```python
from build123d import *

# Parameters (mm, degrees)
BASE_W_MOTOR_MOUNTS_R     = 70
BASE_W_MOTOR_MOUNTS_R_2   = 1.651
BOSS_EXTRUDE1_DEPTH       = 3.175
STANDOFFS_TOP_BOTTOM_R    = 1.65
CUT_EXTRUDE2_DEPTH        = 3.175
PI_AND_MEGA_STANDOFFS_R   = 1.4
PI_AND_MEGA_STANDOFFS_R_2 = 1.65
CUT_EXTRUDE3_DEPTH        = 3.175


with BuildPart() as part:
    # Base w/ Motor Mounts → Boss-Extrude1 (new body)
    with BuildSketch(Plane(origin=(0, 0, 0), x_dir=(1, 0, 0), z_dir=(0, 1, 0))):
        Circle(BASE_W_MOTOR_MOUNTS_R)
        with Locations((44.55, 0)):
            Circle(BASE_W_MOTOR_MOUNTS_R_2, mode=Mode.SUBTRACT)
        with Locations((54.075, 10.85)):
            Circle(BASE_W_MOTOR_MOUNTS_R_2, mode=Mode.SUBTRACT)
        with Locations((54.075, -10.85)):
            Circle(BASE_W_MOTOR_MOUNTS_R_2, mode=Mode.SUBTRACT)
        with Locations((-54.075, -10.85)):
            Circle(BASE_W_MOTOR_MOUNTS_R_2, mode=Mode.SUBTRACT)
        with Locations((-54.075, 10.85)):
            Circle(BASE_W_MOTOR_MOUNTS_R_2, mode=Mode.SUBTRACT)
        with Locations((-44.55, 0)):
            Circle(BASE_W_MOTOR_MOUNTS_R_2, mode=Mode.SUBTRACT)
    extrude(amount=BOSS_EXTRUDE1_DEPTH)

    # Standoffs (top / bottom) → Cut-Extrude2 (cut)
    with BuildSketch(Plane(origin=(0, 0, 0), x_dir=(1, 0, 0), z_dir=(0, 1, 0))):
        with Locations((60.976049146, 25.257106536)):
            Circle(STANDOFFS_TOP_BOTTOM_R)
        with Locations((60.976049146, -25.257106536)):
            Circle(STANDOFFS_TOP_BOTTOM_R)
        with Locations((-60.976049146, -25.257106536)):
            Circle(STANDOFFS_TOP_BOTTOM_R)
        with Locations((-60.976049146, 25.257106536)):
            Circle(STANDOFFS_TOP_BOTTOM_R)
        with Locations((35, 48.621778265)):
            Circle(STANDOFFS_TOP_BOTTOM_R)
        with Locations((35, 30.621778265)):
            Circle(STANDOFFS_TOP_BOTTOM_R)
        with Locations((35, -30.621778265)):
            Circle(STANDOFFS_TOP_BOTTOM_R)
        with Locations((35, -48.621778265)):
            Circle(STANDOFFS_TOP_BOTTOM_R)
        with Locations((-35, -48.621778265)):
            Circle(STANDOFFS_TOP_BOTTOM_R)
        with Locations((-35, -30.621778265)):
            Circle(STANDOFFS_TOP_BOTTOM_R)
        with Locations((-35, 30.621778265)):
            Circle(STANDOFFS_TOP_BOTTOM_R)
        with Locations((-35, 48.621778265)):
            Circle(STANDOFFS_TOP_BOTTOM_R)
    extrude(amount=CUT_EXTRUDE2_DEPTH, mode=Mode.SUBTRACT)

    # Pi and Mega Standoffs → Cut-Extrude3 (cut)
    with BuildSketch(Plane(origin=(0, 0, 0), x_dir=(1, 0, 0), z_dir=(0, 1, 0))):
        with Locations((-19.9, 55)):
            Circle(PI_AND_MEGA_STANDOFFS_R)
        with Locations((38.1, 55)):
            Circle(PI_AND_MEGA_STANDOFFS_R)
        with Locations((38.1, 6)):
            Circle(PI_AND_MEGA_STANDOFFS_R)
        with Locations((-19.9, 6)):
            Circle(PI_AND_MEGA_STANDOFFS_R)
        with Locations((-38.1, -54.2)):
            Circle(PI_AND_MEGA_STANDOFFS_R_2)
        with Locations((-36.8, -6)):
            Circle(PI_AND_MEGA_STANDOFFS_R_2)
        with Locations((38.1, -6)):
            Circle(PI_AND_MEGA_STANDOFFS_R_2)
    extrude(amount=CUT_EXTRUDE3_DEPTH, mode=Mode.SUBTRACT)


solid = part.part
```
Design review of the part built by this model. Coordinates are the model's own, in mm. Coordinates: 2 decimals unless noted, no trailing zeros. Order: outer loops, then holes, each group sorted by start corner. A loop starts at its lowest first (then second) coordinate and runs counter-clockwise, first axis right, second up. Notation, with made-up numbers: M 7,48.25 L 19,48.25 A19 ccw 19,76.25 Z; hole C -23,-11.75 d10. An arc over 180 degrees is marked long. Answer as a JSON object with one key per item and string values. Group by question number.
1) For pin 1 (1 mm diameter, centred on y = 1, z = -53.5, fed in from +X), flat-tipped, find the tip position at first contact; note if it passes through.
2) Wall thickness on L1, parallel to Z at x = -19.9, y = 2.5; L2, parallel to Z at x = -35, y = 1.6; L3, parallel to Z at x = 37, y = 0.9: over which ranges is each line inside the solid? List them lowest first.
3) Add section D-D, the plane x = -24.5. Write out the cut boundary in (y, z) (3 decimals).
4) Add section C-C, the plane x = -44.55. Write out the cut boundary in (y, z) (1 decimal), then the cut area to 3 significant figures.
5) Add section B-B, the plane y = 2.25. Count the separate pieces of the cut face and the enclosed holes in it, then the cut area to 3 significant figures.
6) Mouldability with a two-part tool opening along Z and no side actions: class faces 1 (the flat face through (-1, 0, -1)), 2 (the cylindrical face through (-36.65, 1.57, -48.69)) as pulls with the +Z half, pulls with the -Z half, needs draft (parallel to the pull), parting line crosses it, or undercut.
7) Add section A-A, the plane z = 0. Write out the cut boundary in (x, y) (3 decimals), then the cut area to 3 significant figures.
Computed values:
{
 "1": {"pin 1": "stops at x = 45.73"},
 "2": {"L1": "z = -67.11 to -56.4, -53.6 to -7.4, -4.6 to 67.11", "L2": "z = -60.62 to -50.27, -46.97 to -32.27, -28.97 to 28.97, 32.27 to 46.97, 50.27 to 60.62", "L3": "z = -59.42 to -55.87, -54.13 to -6.87, -5.13 to 4.77, 7.23 to 59.42"},
 "3": {"outline": "M 0,-65.572 L 3.175,-65.572 L 3.175,65.572 L 0,65.572 Z"},
 "4": {"outline": "M 0,-54 L 3.2,-54 L 3.2,-1.7 L 0,-1.7 Z; M 0,1.7 L 3.2,1.7 L 3.2,54 L 0,54 Z", "area": "332 mm^2"},
 "5": {"separate pieces": "1", "enclosed holes": "25", "area": "15,200 mm^2"},
 "6": {"face 1": "needs draft", "face 2": "undercut"},
 "7": {"outline": "M -70,0 L -46.201,0 L -46.201,3.175 L -70,3.175 Z; M -42.899,0 L 42.899,0 L 42.899,3.175 L -42.899,3.175 Z; M 46.201,0 L 70,0 L 70,3.175 L 46.201,3.175 Z", "area": "424 mm^2"}
}
